Read the model definition and answer for the solid it produces. Units are mm, in the model's axes. Face numbers are marked on the shaded views. A direction names the side the tool comes from. Round coordinates to 2 decimals unless told otherwise and drop trailing zeros. Order: outer loops, then holes, each group sorted by start corner. A loop starts at its lowest first (then second) coordinate and runs counter-clockwise, first axis right, second up. Notation, with made-up numbers: M 12,-3.75 L 51,-3.75 A15 cw 51,22.25 Z; hole C -21,17 d6. An arc over 180 degrees is marked long. Answer as CSV lines item,"result".
```python
from build123d import *

# Parameters (mm, degrees)
F1_DEPTH = 25.4
F2_R     = 12.7
F3_DEPTH = 25.4


with BuildPart() as f1:
    # F0 (on Front) → F1 (new body)
    with BuildSketch(Plane.XZ):
        with BuildLine():
            ThreePointArc((-37.03413, 21.034328), (-63.178262, 22.436599), (-76.672003, 0))
            ThreePointArc((-76.672003, 0), (-69.232515, -17.960512), (-51.272003, -25.4))
            ThreePointArc((-51.272003, -25.4), (-33.31149, -17.960512), (-25.872003, 0))
            ThreePointArc((-25.872003, 0), (-28.835403, 11.906259), (-37.03413, 21.034328))
        make_face()
        with BuildLine():
            ThreePointArc((-38.572003, 0), (-42.291747, -8.980256), (-51.272003, -12.7))
            ThreePointArc((-51.272003, -12.7), (-60.252259, 8.980256), (-38.572003, 0))
        make_face(mode=Mode.SUBTRACT)
        with BuildLine():
            Line((-76.672003, 0), (-76.672003, -50.8))
            Line((-76.672003, -50.8), (-51.272003, -50.8))
            Line((-51.272003, -50.8), (-51.272003, -25.4))
            ThreePointArc((-51.272003, -25.4), (-69.232515, -17.960512), (-76.672003, 0))
        make_face()
        with BuildLine():
            Line((-51.272003, -25.4), (-51.272003, -50.8))
            Line((-51.272003, -50.8), (50.327997, -50.8))
            Line((50.327997, -50.8), (50.327997, -38.1))
            Line((50.327997, -38.1), (-37.03413, 21.034328))
            ThreePointArc((-37.03413, 21.034328), (-28.835403, 11.906259), (-25.872003, 0))
            ThreePointArc((-25.872003, 0), (-33.31149, -17.960512), (-51.272003, -25.4))
        make_face()
    extrude(amount=F1_DEPTH)

    # F2 (on face) → F3 (join)
    with BuildSketch(Plane.XZ.offset(25.4)):
        with BuildLine():
            Line((50.327997, -50.8), (50.327997, -38.1))
            Line((50.327997, -38.1), (-25.872003, -38.1))
            Line((-25.872003, -38.1), (-25.872003, 0))
            ThreePointArc((-25.872003, 0), (-28.835403, 11.906259), (-37.03413, 21.034328))
            ThreePointArc((-37.03413, 21.034328), (-63.178262, 22.436599), (-76.672003, 0))
            Line((-76.672003, 0), (-76.672003, -38.1))
            Line((-76.672003, -38.1), (-76.672003, -50.8))
            Line((-76.672003, -50.8), (50.327997, -50.8))
        make_face()
        with Locations((-51.272003, 0)):
            Circle(F2_R, mode=Mode.SUBTRACT)
    extrude(amount=F3_DEPTH)


solid = f1.part
```
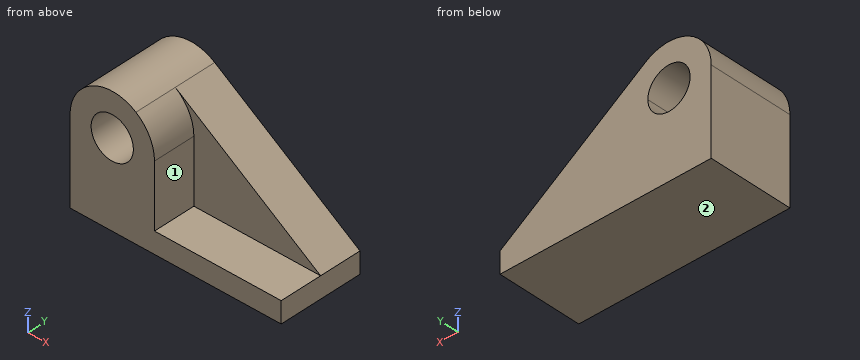
Item 1: A tool of negligible diameter and unlimited length cuts with its end or side. For the marked faces 1 and 2, from which of +Z, -Z, +X, -X, +Y, -Y can it reach the whole face along a straight path? Write none if from no direction.
Ans:
face 1,"+Z, +X, -Y"
face 2,"-Z, +X, -X, +Y, -Y"
Item 2: A cutting plane is placed at B-B, the plane z = 8.5. Determine the outline of the cut face in (x, y).
Ans:
outline,"M -75.21,-50.8 L -60.71,-50.8 L -60.71,0 L -75.21,0 Z; M -41.84,-50.8 L -27.34,-50.8 L -27.34,-25.4 L -18.52,-25.4 L -18.52,0 L -41.84,0 Z"
Item 3: A cutting plane is placed at D-D, the plane x = -8. Determine the outline of the cut face in (y, z), and give its area (3 significant figures).
Ans:
outline,"M -50.8,-50.8 L 0,-50.8 L 0,1.38 L -25.4,1.38 L -25.4,-38.1 L -50.8,-38.1 Z"
area,"1,650 mm2"
Item 4: A cutting plane is placed at A-A, the plane y = -16. Determine the outline of the cut face in (x, z), and give its area (3 significant figures).
Ans:
outline,"M -76.67,-50.8 L 50.33,-50.8 L 50.33,-38.1 L -37.03,21.03 A25.4 ccw -76.67,0 Z; hole C -51.27,0 d25.4"
area,"6,050 mm2"
Item 5: Find the intervals of material crossed by probe 1 along X at (y, z) = (-31.5, 0); probe 2 along X at (y, z) = (-31.5, -23.5); probe 3 along X at (y, z) = (-39, 4), in increasing order. Write a range as [from, to].
Ans:
probe 1,"[-76.67, -63.97], [-38.57, -25.87]"
probe 2,"[-76.67, -25.87]"
probe 3,"[-76.36, -63.33], [-39.22, -26.19]"
Item 6: Flat-ended cylindrical pins translate along their axes: pin 1 (20.5 mm diameter, centred on x = 4, y = -42.5, fed in from +Z); pin 2 (10 mm diameter, centred on y = -13, z = 17.5, fed in from +X); pin 3 (8 mm diameter, centred on y = -6.5, z = 11, fed in from +X). Find the tip coordinate at first contact, or state that the pin passes through.
Ans:
pin 1,"z = -38.1"
pin 2,"x = -24.43"
pin 3,"x = -16.3"
Item 7: A cutting plane is placed at C-C, the plane z = -27. Determine the outline of the cut face in (x, y).
Ans:
outline,"M -76.67,-50.8 L -25.87,-50.8 L -25.87,-25.4 L 33.93,-25.4 L 33.93,0 L -76.67,0 Z"
